Geometry: final body of the model. Coordinates: model frame, mm. Face numbers are marked on the shaded views. Coordinates: 2 decimals unless noted, no trailing zeros. Loops run counter-clockwise (first coordinate to the right, second up) from the corner with the lowest first, then second, coordinate; pieces in that order, holes last. Notation, with made-up numbers: (77, 80) -> (135, 80) arc R12 ccw to (135, 85) -> close; hole circle Ø8 at (70.5, 59.5). An arc over 180 degrees is marked (long way). One line per item, written item: value. Start each with the question number.
Item 1: Ray query, probe 1 along X at (y, z) = (1.5, -53.5); probe 2 along X at (y, z) = (5, -51.25); probe 3 along Y at (x, z) = (38, -53). Return the intervals inside material, ascending. Write a range as from..to.
Item 2: Section query C-C on y = 15.75. Return loops of the section in (x, z).
Item 3: Section query B-B on x = 20.5. Return loops of the section in (y, z).
Item 4: Section query A-A on y = 12.5. Return loops of the section in (x, z), then the cut area to 3 significant figures.
Item 5: Mould query, pull axis X, two halves, no side actions, for the marked faces 1, 2, 3 and 4. Classes: +X half, -X half, draft (parallel to the pull), parting line (faces both ways), or undercut.
Item 6: Section query D-D on y = -0.5. Return loops of the section in (x, z).
Item 7: Contact query for flat-ended pins moving along their axis: pin 1 Ø1.7 at (y, z) = (2.5, -54.5) entering from +X; pin 2 Ø4 at (x, z) = (43, -52) entering from -Y; pin 3 Ø1 at (y, z) = (12.5, -53) entering from +X; pin 4 Ø1.6 at (y, z) = (-0.5, -55) entering from -X (3 decimals). Output: stop coordinate, or through.
from build123d import *

# Parameters (mm, degrees)
BOSS_EXTRUDE3_DEPTH = 6.5
BOSS_EXTRUDE4_DEPTH = 7.8
CHAMFER1_SIZE       = 1
FILLET1_R           = 2


with BuildPart() as part:
    # Sketch2 → Boss-Extrude3 (new body)
    with BuildSketch(Plane(origin=(0, 0, 0), x_dir=(1, 0, 0), z_dir=(0, 1, 0))):
        Polygon((30.214970749, 56.232123089), (30.214970749, 50.432123089), (17.514970749, 50.432123089), (17.514970749, 56.232123089), (19.514970749, 56.232123089), (19.514970749, 57.232123089), (16.514970749, 57.232123089), (16.514970749, 49.432123089), (31.214970749, 49.432123089), (31.214970749, 57.232123089), (28.214970749, 57.232123089), (28.214970749, 56.232123089), align=None)
    extrude(amount=BOSS_EXTRUDE3_DEPTH)

    # Sketch1 → Boss-Extrude4 (add)
    with BuildSketch(Plane(origin=(-49.432123089, 0, -49.432123089), x_dir=(1, 0, 0), z_dir=(0, 0, 1))):
        Polygon((82.376068434, 3.015544457), (81.2123933, 1), (80.647093838, 1), (80.647093838, 0), (81.367093838, 0), (81.367093838, -1.41), (79.367093838, -1.41), (79.367093838, -2.41), (82.367093838, -2.41), (82.367093838, 1), (83.742093838, 3.38156986), (82.578418703, 4.053418013), (83.742093838, 6.068962469), (82.578418703, 6.740810621), (83.742093838, 8.756355078), (82.578418703, 9.42820323), (83.742093838, 11.443747687), (82.578418703, 12.115595839), (83.742093838, 14.131140296), (82.578418703, 14.802988448), (83.742093838, 16.818532905), (83.2123933, 17.124355653), (105.2123933, 17.124355653), (105.2123933, 23.124355653), (70.647093838, 23.124355653), (70.647093838, 7.499909308), (78.647093838, 6.8), (78.647093838, 17.124355653), (81.2123933, 17.124355653), (82.376068434, 16.452507501), (81.2123933, 14.436963044), (82.376068434, 13.765114892), (81.2123933, 11.749570435), (82.376068434, 11.077722283), (81.2123933, 9.062177826), (82.376068434, 8.390329674), (81.2123933, 6.374785218), (82.376068434, 5.702937065), (81.2123933, 3.687392609), align=None)
    extrude(amount=-BOSS_EXTRUDE4_DEPTH)

    # Chamfer1
    chamfer1_edges = [part.edges().sort_by_distance(p)[0] for p in [
        (29.214970749, 11.962177826, -49.432123089),
        (21.214970749, 15.312132481, -49.432123089),
        (55.780270211, 20.124355653, -49.432123089),
        (29.214970749, 11.962177826, -57.232123089),
        (21.214970749, 15.312132481, -57.232123089),
        (55.780270211, 20.124355653, -57.232123089),
    ]]
    chamfer(chamfer1_edges, length=CHAMFER1_SIZE)

    # Fillet1
    fillet1_edges = [part.edges().sort_by_distance(p)[0] for p in [
        (29.214970749, 6.8, -53.332123089),
        (29.214970749, 17.124355653, -53.332123089),
        (21.214970749, 7.499909308, -53.332123089),
        (21.214970749, 23.124355653, -53.332123089),
        (55.780270211, 17.124355653, -53.332123089),
        (55.780270211, 23.124355653, -53.332123089),
    ]]
    fillet(fillet1_edges, radius=FILLET1_R)


solid = part.part
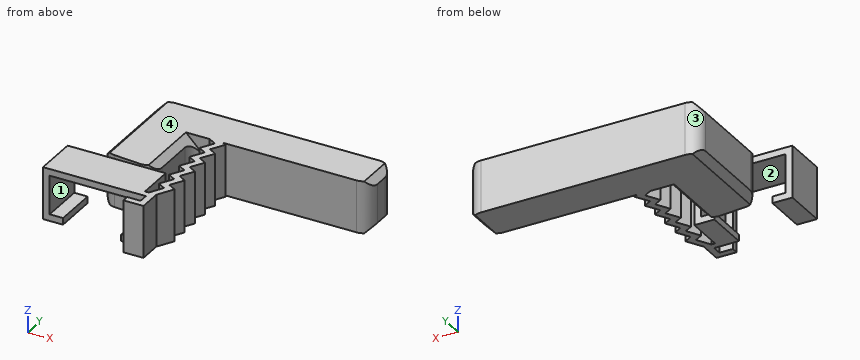
Reply:
1. probe 1: x = 16.51..17.51, 30.21..31.21, 32.07..33.22
1. probe 2: x = 16.51..17.51, 30.21..31.21, 32.54..33.69
1. probe 3: y = 17.12..23.12
2. outline: (21.21, -56.23) -> (22.21, -57.23) -> (28.21, -57.23) -> (29.32, -56.13) -> (29.32, -50.53) -> (28.21, -49.43) -> (22.21, -49.43) -> (21.21, -50.43) -> close; (32.54, -57.23) -> (33.69, -57.23) -> (33.69, -49.43) -> (32.54, -49.43) -> close
3. outline: (0, -50.43) -> (6.5, -50.43) -> (6.5, -49.43) -> (0, -49.43) -> close
4. outline: (21.21, -56.23) -> (22.21, -57.23) -> (28.21, -57.23) -> (29.21, -56.23) -> (29.21, -50.43) -> (28.21, -49.43) -> (22.21, -49.43) -> (21.21, -50.43) -> close; (32.21, -57.23) -> (33.37, -57.23) -> (33.37, -49.43) -> (32.21, -49.43) -> close
4. area: 69.4 mm²
5. face 1: undercut
5. face 2: undercut
5. face 3: -X half
5. face 4: draft
6. outline: (31.93, -57.23) -> (32.93, -57.23) -> (32.93, -49.43) -> (31.93, -49.43) -> close
7. pin 1: stops at x = 34.29
7. pin 2: stops at y = 17.12
7. pin 3: stops at x = 33.66
7. pin 4: stops at x = 16.515
